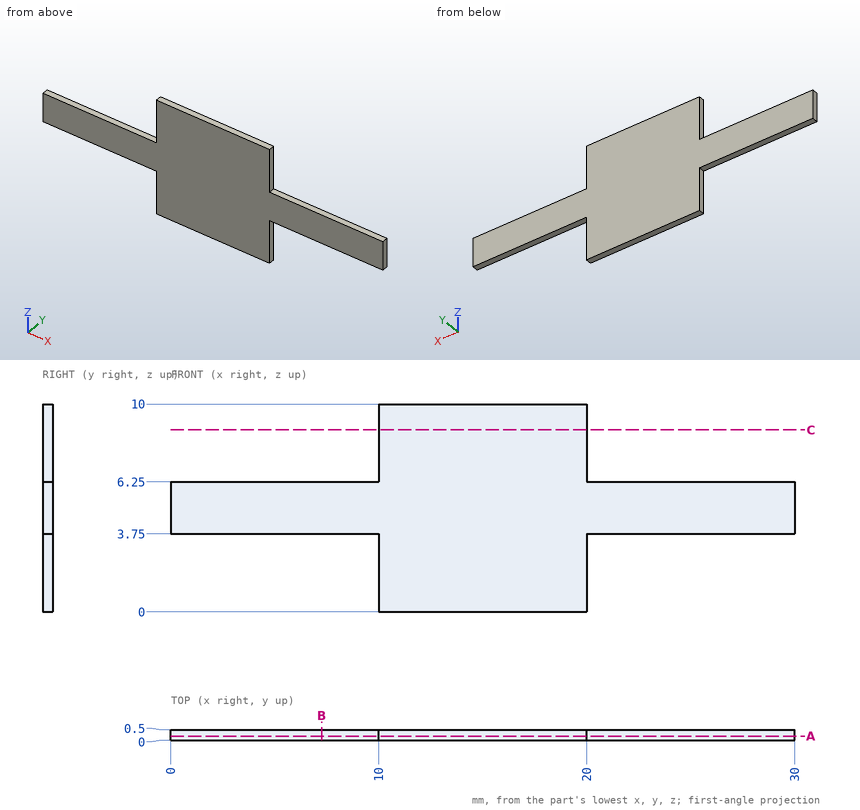
Could you check a few things on this drawing? It's one solid part, dimensions in mm from its lowest x, y, z. Give positions to 0.01 mm unless a question says otherwise; leave off trailing zeros. Loops run counter-clockwise (first coordinate to the right, second up) from the corner with the lowest first, then second, coordinate; pieces in that order, holes last. Notation, with made-up numbers: (72.5, 42.25) -> (131.5, 42.25) arc R33 ccw to (131.5, 70.25) -> close; hole circle Ø5 at (-15, 43). An arc over 180 degrees is marked (long way). Use one line per item in the form item = value. Start each with the question number.
1) Imagine slicing it at B-B (x = 7.25). Please give me the cut outline in (y, z).
2) Please list where these lines run through material, in increasing order: line 1 along X through (y, z) = (0.4, 2.25); line 2 along Z through (x, y) = (24, 0.15).
3) For P1, Ø1.5, axis at x = 16.5, z = 2.5, coming from the -Y side, with a flat end and sliding along its axis, tell me the tip position at first contact or that it passes through.
4) Imagine slicing it at C-C (z = 8.75). Please give me the cut outline in (x, y).
5) Imagine slicing it at A-A (y = 0.2). Please give me the cut outline in (x, z), then the cut area to 3 significant figures.
Check values:
q1.outline = (0, 3.75) -> (0.5, 3.75) -> (0.5, 6.25) -> (0, 6.25) -> close
q2.line_1 = 10 to 20
q2.line_2 = 3.75 to 6.25
q3.P1 = 0
q4.outline = (10, 0) -> (20, 0) -> (20, 0.5) -> (10, 0.5) -> close
q5.outline = (0, 3.75) -> (10, 3.75) -> (10, 0) -> (20, 0) -> (20, 3.75) -> (30, 3.75) -> (30, 6.25) -> (20, 6.25) -> (20, 10) -> (10, 10) -> (10, 6.25) -> (0, 6.25) -> close
q5.area = 150 mm^2
